Geometry check sheet. Reference: the model listing, model coordinates, mm. A direction names the side the tool comes from. Round coordinates to 2 decimals unless told otherwise and drop trailing zeros. Write each loop counter-clockwise with the first axis right and the second up, starting at its lowest first coordinate (ties: lowest second). Pieces come first, ordered by that corner, then holes. Notation, with made-up numbers: M 33.5,-12.5 L 43.5,-12.5 A27 ccw 43.5,11.5 Z; hole C 58,1 d6. An arc over 180 degrees is marked long. Answer in a Markdown table with one row per item. Add a question column.
from build123d import *

# Parameters (mm, degrees)
BOSS_EXTRUDE1_DEPTH = 10.16
CUT_EXTRUDE1_DEPTH  = 1.27
FILLET2_R           = 1.27
FILLET3_R           = 1.27


with BuildPart() as part:
    # Sketch1 → Boss-Extrude1 (new body)
    with BuildSketch(Plane(origin=(0, 0, 0), x_dir=(1, 0, 0), z_dir=(0, 1, 0))):
        with BuildLine():
            Line((0, 3.81), (15.24, 3.81))
            ThreePointArc((15.24, 3.81), (19.05, 0), (15.24, -3.81))
            Line((15.24, -3.81), (0, -3.81))
            ThreePointArc((0, -3.81), (-3.81, 0), (0, 3.81))
        make_face()
    extrude(amount=BOSS_EXTRUDE1_DEPTH)

    # Sketch2 → Cut-Extrude1 (cut)
    with BuildSketch(Plane(origin=(0, 10.16, 0), x_dir=(1, 0, 0), z_dir=(0, 1, 0))):
        Polygon((2.748829604, -0.902510302), (2.748829604, 0.902510302), (8.660197845, 0.902510302), (8.660197845, 2.14567358), (13.937299107, 0), (8.660197845, -2.14567358), (8.660197845, -0.902510302), align=None)
    extrude(amount=-CUT_EXTRUDE1_DEPTH, mode=Mode.SUBTRACT)

    # Fillet2
    fillet2_edges = [part.edges().sort_by_distance(p)[0] for p in [
        (19.05, 10.16, 0),
        (7.62, 10.16, -3.81),
        (-3.81, 10.16, 0),
        (7.62, 10.16, 3.81),
    ]]
    fillet(fillet2_edges, radius=FILLET2_R)

    # Fillet3
    fillet3_edges = [part.edges().sort_by_distance(p)[0] for p in [
        (7.62, 0, -3.81),
        (19.05, 0, 0),
        (7.62, 0, 3.81),
        (-3.81, 0, 0),
    ]]
    fillet(fillet3_edges, radius=FILLET3_R)


solid = part.part
Item 1: Section check A-A, the plane x = 6.25. Record the boundary of the cut face in (y, z), and give its area (3 significant figures).
Item 2: Access from +Z, -Z, +X, -X, +Y, -Y to the whole of each face (thin tool, end or side, straight path). Record for faces 5 (the flat face through (8.66, 9.5, 1.5)), 6 (the cylindrical face through (7.727, 0.382, -3.448)).
Item 3: Mould release check, pull along Z, two halves, no side actions. Record for faces 1 (the flat face through (8, 0, 0)), 2 (the flat face through (8, 5, 3.81)), 3 (the cylindrical face through (-3.81, 5.03, 0.08)), 4 (the flat face through (8.66, 9.5, -1.5)): +Z half, -Z half, draft (parallel to the pull), parting line (faces both ways), or undercut.
Item 4: Section check B-B, the plane y = 6. Record the boundary of the cut face in (x, z), and give its area (3 significant figures).
Item 5: Scan lines: probe 1 along Z at (x, y) = (10.25, 9.5); probe 2 along Y at (x, z) = (10.5, 0.5); probe 3 along X at (y, z) = (9, 2). Record each from-to range of solid material in increasing order. Write a range as from..to.
Item 6: Gauge pin test, flat ends, axial feed: pin 1 Ø1.4 at (y, z) = (10, 0.5) entering from +X; pin 2 Ø1 at (x, y) = (6, 9.5) entering from +Z; pin 3 Ø1 at (x, z) = (9.5, 0.5) entering from +Y. Record the tip position at first contact, or that the pin passes through.
Result sheet:
| question | item | result |
|---|---|---|
| 1 | outline | M 0,-2.54 A1.27 ccw 1.27,-3.81 L 8.89,-3.81 A1.27 ccw 10.16,-2.54 L 10.16,-0.9 L 8.89,-0.9 L 8.89,0.9 L 10.16,0.9 L 10.16,2.54 A1.27 ccw 8.89,3.81 L 1.27,3.81 A1.27 ccw 0,2.54 Z |
| 1 | area | 73.7 mm^2 |
| 2 | face 5 | +Y |
| 2 | face 6 | -Z, +X, -X, -Y |
| 3 | face 1 | draft |
| 3 | face 2 | +Z half |
| 3 | face 3 | parting line |
| 3 | face 4 | undercut |
| 4 | outline | M 0,-3.81 L 15.24,-3.81 A3.81 ccw 15.24,3.81 L 0,3.81 A3.81 ccw Z |
| 4 | area | 162 mm^2 |
| 5 | probe 1 | z = -3.65..-1.5, 1.5..3.65 |
| 5 | probe 2 | y = 0..8.89 |
| 5 | probe 3 | x = -3.24..8.66, 9.02..18.48 |
| 6 | pin 1 | stops at x = 18.96 |
| 6 | pin 2 | stops at z = 3.81 |
| 6 | pin 3 | stops at y = 8.89 |
